The listing builds one solid part. Answer for the finished solid, in the listing's coordinates (mm). A direction names the side the tool comes from. Round coordinates to 2 decimals unless told otherwise and drop trailing zeros. Order: outer loops, then holes, each group sorted by start corner. A loop starts at its lowest first (then second) coordinate and runs counter-clockwise, first axis right, second up. Notation, with made-up numbers: (-27, -6) -> (21, -6) arc R20 cw to (21, 22) -> close; hole circle Ø1 at (-38.5, 46). An arc over 180 degrees is marked (long way). Return JSON: item names as keys, results as strings. Group by question number.
(1) The part is cut by section C-C (z = 50). Determine the outline of the cut face in (x, y) (3 decimals), plus the area to 3 significant figures.
(2) The part is cut by section B-B (x = -17.5). Determine the outline of the cut face in (y, z) (3 decimals), plus the area to 3 significant figures.
(3) Determine the mould class of faces 3 (the face through (0, -9.525, 1)), 4 (the face through (0, 3, -73.025)), 5 (the face through (-21.59, 8, -1)) for opening direction Z: +Z half, -Z half, draft (parallel to the pull), parting line (faces both ways), or undercut.
(4) Consider line 1 (Z direction, x = 0, y = 9.25) (3 decimals); line 2 (X direction, y = 4, z = 56) (3 decimals); line 3 (Y direction, x = 9, z = 34.5) (3 decimals). Determine where each line is inside the solid, lowest interval first. Write a range as [from, to].
(5) This flat-tipped pin is pushed along its axis until it touches: pin 1 (21.5 mm diameter, centred on x = -0.5, z = 5, fed in from +Y). Where does it stop, or does it pass through?
(6) The part is cut by section A-A (y = 10.75). Determine the outline of the cut face in (x, z) (3 decimals).
(7) Which of the six approach directions +Z, -Z, +X, -X, +Y, -Y give full straight-line access (tool end or side, diameter ignored) to faces 1 (the face through (21.59, 8, 1)), 2 (the face through (31.115, 3, 1))?
Autodesk Inventor part; units mm, degrees
ref_plane "XZ Plane" through (0, 0, 0) normal (0, 1, 0) x (-1, 0, 0)
ref_plane "XY Plane" through (0, 0, 0) normal (0, 0, 1) x (1, 0, 0)
sketch "Sketch1" plane through (0, 0, 0) normal (0, 1, 0) x (-1, 0, 0)
  line L0 (31.115, 73.025) -> (-31.115, 73.025)
  line L1 (-31.115, 73.025) -> (-31.115, -73.025)
  line L2 (-31.115, -73.025) -> (31.115, -73.025)
  line L3 (31.115, -73.025) -> (31.115, 73.025)
  line L4 (31.115, 73.025) -> (-31.115, -73.025) construction
  line L5 (-31.115, 73.025) -> (31.115, -73.025) construction
  point P0 (0, 0)
  dimension "outerWidth" = 62.23
  dimension "outerLength" = 146.05
extrude "Extrusion1" add sketch "Sketch1" against normal blind 9.525
sketch "Sketch2" plane through (0, 0, 0) normal (0, 1, 0) x (1, 0, 0)
  line L0 (31.115, -73.025) -> (31.115, 73.025)
  line L1 (31.115, 73.025) -> (-31.115, 73.025)
  line L2 (-31.115, 73.025) -> (-31.115, -73.025)
  line L3 (-31.115, -73.025) -> (31.115, -73.025)
  line L4 (31.115, -73.025) -> (-31.115, 73.025) construction
  line L5 (31.115, 73.025) -> (-31.115, -73.025) construction
  line L6 (21.59, -63.5) -> (21.59, 63.5)
  line L7 (21.59, 63.5) -> (-21.59, 63.5)
  line L8 (-21.59, 63.5) -> (-21.59, -63.5)
  line L9 (-21.59, -63.5) -> (21.59, -63.5)
  line L10 (21.59, -63.5) -> (-21.59, 63.5) construction
  line L11 (21.59, 63.5) -> (-21.59, -63.5) construction
  line L12 (31.115, 73.025) -> (-31.115, 73.025)
  line L13 (-31.115, 73.025) -> (-31.115, -73.025)
  point P0 (0, 0)
  dimension "d1" = 9.525
  dimension "d5" = 9.525
extrude "Extrusion2" add sketch "Sketch2" along normal blind 15.875
equation "\"outerWidth\" = innerWidth + 2 * wallThickness"
equation "\"outerLength\" = innerLength + 2 * wallThickness"
equation "\"d2\" = wallThickness"
equation "\"d1\" = wallThickness"
equation "\"d5\" = wallThickness"
equation "\"d4\" = outerHeight - wallThickness"
equation "\"innerLength\" = 127"
equation "\"width\" = 196.85"
equation "\"outerHeight\" = 25.4"
equation "\"wallThickness\" = 9.525"
properties part number "connectorToTubeBrackets" material "PC/ABS Plastic"
Answer below:
{
 "1": {"outline": "(-31.115, -9.525) -> (31.115, -9.525) -> (31.115, 15.875) -> (21.59, 15.875) -> (21.59, 0) -> (-21.59, 0) -> (-21.59, 15.875) -> (-31.115, 15.875) -> close", "area": "895 mm²"},
 "2": {"outline": "(-9.525, -73.025) -> (15.875, -73.025) -> (15.875, -63.5) -> (0, -63.5) -> (0, 63.5) -> (15.875, 63.5) -> (15.875, 73.025) -> (-9.525, 73.025) -> close", "area": "1,690 mm²"},
 "3": {"face 3": "draft", "face 4": "-Z half", "face 5": "undercut"},
 "4": {"line 1": "z = [-73.025, -63.5], [63.5, 73.025]", "line 2": "x = [-31.115, -21.59], [21.59, 31.115]", "line 3": "y = [-9.525, 0]"},
 "5": {"pin 1": "stops at y = 0"},
 "6": {"outline": "(-31.115, -73.025) -> (31.115, -73.025) -> (31.115, 73.025) -> (-31.115, 73.025) -> close; hole (-21.59, -63.5) -> (21.59, -63.5) -> (21.59, 63.5) -> (-21.59, 63.5) -> close"},
 "7": {"face 1": "+Y", "face 2": "+Z, -Z, +X, +Y, -Y"}
}
